Here's the drawing with two shaded views (mm, measured from the low corner). I have some questions. Coordinates: 2 decimals unless noted, no trailing zeros. Write each loop counter-clockwise with the first axis right and the second up, starting at its lowest first coordinate (ties: lowest second). Pieces come first, ordered by that corner, then holes.
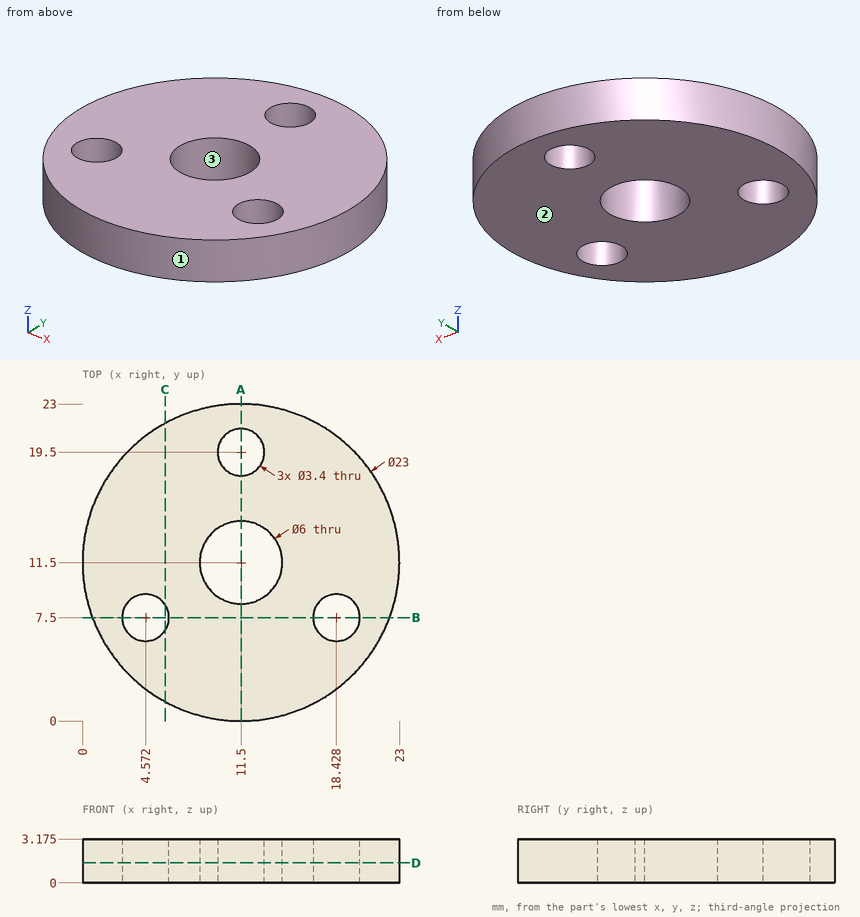
1. If we mould it in two halves opening along X, with no side actions, what happens to the marked faces 1, 2 and 3? For each: pulls with the +X half, pulls with the -X half, needs draft (parallel to the pull), parting line crosses it, or undercut.
Verdict:
face 1: parting line crosses it
face 2: needs draft
face 3: undercut
2. I want a section at D-D on z = 1.45. Please give me the cut outline in (x, y), plus the area to 3 significant figures.
Verdict:
outline: circle Ø23 at (11.5, 11.5); hole circle Ø3.4 at (4.57, 7.5); hole circle Ø6 at (11.5, 11.5); hole circle Ø3.4 at (11.5, 19.5); hole circle Ø3.4 at (18.43, 7.5)
area: 360 mm2
3. I want a section at C-C on x = 6. Please give me the cut outline in (y, z) (1 decimal), plus the area to 3 significant figures.
Verdict:
outline: (1.4, 0) - (6.6, 0) - (6.6, 3.2) - (1.4, 3.2) - close; (8.4, 0) - (21.6, 0) - (21.6, 3.2) - (8.4, 3.2) - close
area: 58.3 mm2
4. Please list where these lines run through material, in increasing order: line 1 along Y through (x, z) = (11.5, 0.9); line 2 along X through (y, z) = (8.25, 3.05); line 3 along Y through (x, z) = (8.75, 0.6) (1 decimal).
Verdict:
line 1: y = 0 to 8.5, 14.5 to 17.8, 21.2 to 23
line 2: x = 0.47 to 3.05, 6.1 to 16.9, 19.95 to 22.53
line 3: y = 0.3 to 10.3, 12.7 to 22.7
5. I want a section at B-B on y = 7.5. Please give me the cut outline in (x, z) (1 decimal).
Verdict:
outline: (0.7, 0) - (2.9, 0) - (2.9, 3.2) - (0.7, 3.2) - close; (6.3, 0) - (16.7, 0) - (16.7, 3.2) - (6.3, 3.2) - close; (20.1, 0) - (22.3, 0) - (22.3, 3.2) - (20.1, 3.2) - close
6. For pin 1 (5.5 mm diameter, centred on x = 18.43, y = 7.5, fed in from +Z) (3 decimals); pin 2 (1 mm diameter, centred on y = 18, z = 1.5, fed in from -X), each with a flat end and sliding along its axis, tell me the tip position at first contact or that it passes through.
Verdict:
pin 1: stops at z = 3.175
pin 2: stops at x = 1.69
7. I want a section at A-A on x = 11.5. Please give me the cut outline in (y, z) (3 decimals), plus the area to 3 significant figures.
Verdict:
outline: (0, 0) - (8.5, 0) - (8.5, 3.175) - (0, 3.175) - close; (14.5, 0) - (17.8, 0) - (17.8, 3.175) - (14.5, 3.175) - close; (21.2, 0) - (23, 0) - (23, 3.175) - (21.2, 3.175) - close
area: 43.2 mm2
